CAD build for the part. Positions are in the model's coordinates, mm. A direction names the side the tool comes from. Give positions to 0.01 mm unless a question says otherwise; leave off trailing zeros. Write each loop counter-clockwise with the first axis right and the second up, starting at its lowest first coordinate (ties: lowest second). Pieces come first, ordered by that corner, then holes. Notation, with made-up numbers: (61, -5.75) -> (70, -5.75) arc R15 ccw to (70, 17.25) -> close; hole circle Ø5 at (-21.75, 71.5). An arc over 180 degrees is marked (long way). Answer as a JSON object with one key per item and string values.
```python
from build123d import *

# Parameters (mm, degrees)
BOSS_EXTRUDE1_DEPTH = 12
FILLET1_R           = 1
SKETCH2_W           = 18.269103957
SKETCH2_H           = 8.189598326
BOSS_EXTRUDE2_DEPTH = 2
BOSS_EXTRUDE2_TAPER = 15
SKETCH4_W           = 17.197307187
SKETCH4_H           = 7.117801556
BOSS_EXTRUDE3_DEPTH = 30
SKETCH5_R           = 2.5
CUT_EXTRUDE1_DEPTH  = 8
SKETCH6_R           = 8.598653593
BOSS_EXTRUDE4_DEPTH = 20
SKETCH7_R           = 7
SKETCH7_R_2         = 3.99890548
CUT_EXTRUDE2_DEPTH  = 5
SKETCH8_R           = 3.99890548
CUT_EXTRUDE3_DEPTH  = 71.566063032


with BuildPart() as part:
    # Sketch1 → Boss-Extrude1 (new body)
    with BuildSketch(Plane(origin=(0, 0, 0), x_dir=(1, 0, 0), z_dir=(0, 1, 0))):
        Polygon((0, -38), (7.071067812, -45.071067812), (33.071067812, -45.071067812), (40.142135624, -38), (40.142135624, 0), (0, 0), align=None)
    extrude(amount=BOSS_EXTRUDE1_DEPTH)

    # Fillet1
    fillet1_edges = [part.edges().sort_by_distance(p)[0] for p in [
        (20.071067812, 12, 45.071067812),
        (36.606601718, 12, 41.535533906),
        (40.142135624, 12, 19),
        (20.071067812, 12, 0),
        (0, 12, 19),
        (3.535533906, 12, 41.535533906),
    ]]
    fillet(fillet1_edges, radius=FILLET1_R)

    # Sketch2 → Boss-Extrude2 (add)
    with BuildSketch(Plane(origin=(0, 12, 0), x_dir=(1, 0, 0), z_dir=(0, 1, 0))):
        with Locations((20.14981395, -8.08561763)):
            Rectangle(SKETCH2_W, SKETCH2_H)
    extrude(amount=BOSS_EXTRUDE2_DEPTH, taper=BOSS_EXTRUDE2_TAPER)

    # Sketch4 → Boss-Extrude3 (add)
    with BuildSketch(Plane(origin=(0, 14, 0), x_dir=(1, 0, 0), z_dir=(0, 1, 0))):
        with Locations((20.14981395, -8.08561763)):
            Rectangle(SKETCH4_W, SKETCH4_H)
    extrude(amount=BOSS_EXTRUDE3_DEPTH)

    # Sketch5 → Cut-Extrude1 (cut)
    with BuildSketch(Plane(origin=(0, 12, 0), x_dir=(1, 0, 0), z_dir=(0, 1, 0))):
        with Locations(Location((33.071067812, -39, 0), (0, 0, 270))):
            Circle(SKETCH5_R)
        with Locations(Location((7.071067812, -39, 0), (0, 0, 270))):
            Circle(SKETCH5_R)
    extrude(amount=-CUT_EXTRUDE1_DEPTH, mode=Mode.SUBTRACT)

    # Sketch6 → Boss-Extrude4 (add)
    with BuildSketch(Plane(origin=(0, 0, 4.526716852), x_dir=(-1, 0, 0), z_dir=(0, 0, -1))):
        with Locations((-20.14981395, 44)):
            Circle(SKETCH6_R)
    extrude(amount=-BOSS_EXTRUDE4_DEPTH)

    # Sketch7 → Cut-Extrude2 (cut)
    with BuildSketch(Plane.XY.offset(24.526716852)):
        with Locations((20.155228961, 43.666817717)):
            Circle(SKETCH7_R)
        with Locations((20.155228961, 43.666817717)):
            Circle(SKETCH7_R_2, mode=Mode.SUBTRACT)
    extrude(amount=-CUT_EXTRUDE2_DEPTH, mode=Mode.SUBTRACT)

    # Sketch8 → Cut-Extrude3 (cut, through all)
    with BuildSketch(Plane.XY.offset(24.526716852)):
        with Locations((20.155228961, 43.666817717)):
            Circle(SKETCH8_R)
    extrude(amount=-CUT_EXTRUDE3_DEPTH, mode=Mode.SUBTRACT)


solid = part.part
```
1) Slice it at C-C (y = 23.5). List the corners of the cut face in (x, z), then the cut area to 3 significant figures.
Model answer:
{"outline": "(11.55, 4.53) -> (28.75, 4.53) -> (28.75, 11.64) -> (11.55, 11.64) -> close", "area": "122 mm2"}
2) Slice it at A-A (z = 14.5). List the corners of the cut face in (x, y), then the cut area to 3 significant figures.
Model answer:
{"outline": "(0, 0) -> (40.14, 0) -> (40.14, 11) arc R1 ccw to (39.14, 12) -> (1, 12) arc R1 ccw to (0, 11) -> close; circle Ø17.2 at (20.15, 44); hole circle Ø8 at (20.16, 43.67)", "area": "663 mm2"}
3) Pin check, flat tips, straight feed: pin 1 (2 mm diameter, centred on y = 30.5, z = 11.5, fed in from -X); pin 2 (8 mm diameter, centred on x = 34, z = 25, fed in from +Y); pin 3 (18 mm diameter, centred on x = 20.16, y = 43.67, fed in from +Z); pin 4 (7 mm diameter, centred on x = 20.16, y = 43.67, fed in from +Z). Stop position of each tip, or through.
Model answer:
{"pin 1": "stops at x = 11.55", "pin 2": "stops at y = 12", "pin 3": "stops at z = 24.53", "pin 4": "passes through"}
4) Wall check: probe 1 along X at (y, z) = (6.5, 39); probe 2 along Z at (x, y) = (17.5, 31); probe 3 along Y at (x, z) = (23, 25). Give the ranges that are in metal, low to high.
Model answer:
{"probe 1": "x = 1 to 4.57, 9.57 to 30.57, 35.57 to 39.14", "probe 2": "z = 4.53 to 11.64", "probe 3": "y = 0 to 12"}
5) 3-axis set-ups, long thin cutter, end or side, ignore diameter. For faces 4 (the cylindrical face through (26.83, 45.77, 22.06)), 5 (the cylindrical face through (6.11, 8.06, 41.31)), 6 (the flat face through (17.6, 50.4, 24.527)), 7 (the flat face through (20, 33, 4.527)): which of +Z, -Z, +X, -X, +Y, -Y reach the whole face in a straight line?
Model answer:
{"face 4": "+Z", "face 5": "+Y", "face 6": "+Z, +X, -X, +Y", "face 7": "-Z, +X, -X, +Y"}
6) Mould opens along Y. For faces 1 (the flat face through (40.142, 5, 19)), 2 (the cylindrical face through (3.787, 11.699, 41.383)), 3 (the flat face through (20, 25, 11.645)) say: released by +Y, released by -Y, zero draft, split by the parting line, or undercut.
Model answer:
{"face 1": "zero draft", "face 2": "released by +Y", "face 3": "undercut"}
7) Slice it at B-B (z = 28). List the corners of the cut face in (x, y), then the cut area to 3 significant figures.
Model answer:
{"outline": "(0, 0) -> (40.14, 0) -> (40.14, 11) arc R1 ccw to (39.14, 12) -> (1, 12) arc R1 ccw to (0, 11) -> close", "area": "481 mm2"}
